Autodesk Inventor part; units mm, degrees
ref_plane "YZ Plane" through (0, 0, 0) normal (1, 0, 0) x (0, 1, 0)
ref_plane "XZ Plane" through (0, 0, 0) normal (0, 1, 0) x (-1, 0, 0)
ref_plane "XY Plane" through (0, 0, 0) normal (0, 0, 1) x (1, 0, 0)
sketch "Sketch1" plane through (0, 0, 0) normal (1, 0, 0) x (0, 1, 0)
  arc A0 (-3.4223, -4.604) -> (-3.4223, -18.104) centre (2.5306, -11.354) ccw
  line L0 (-20.4694, -3.1126) -> (-20.4694, -19.5954)
  line L1 (-3.4223, -18.104) -> (-20.4694, -19.5954)
  line L2 (-3.4223, -4.604) -> (-20.4694, -3.1126)
  point P0 (0, 0)
  dimension "d5" = 23
  dimension "d21" = 9
  dimension "d28" = 85
extrude "Extrusion1" add sketch "Sketch1" along normal blind 14
draft "FaceDraft3" angle 8 pull direction (0, 1, 0) faces at (0, -15.7807, -10.9914) fixed edges at (0, -20.4694, -11.354)
draft "FaceDraft4" angle 8 pull direction (0, 1, 0) faces at (14, -15.7807, -10.9914) fixed edges at (14, -20.4694, -11.354)
properties part number "BaseGarra"
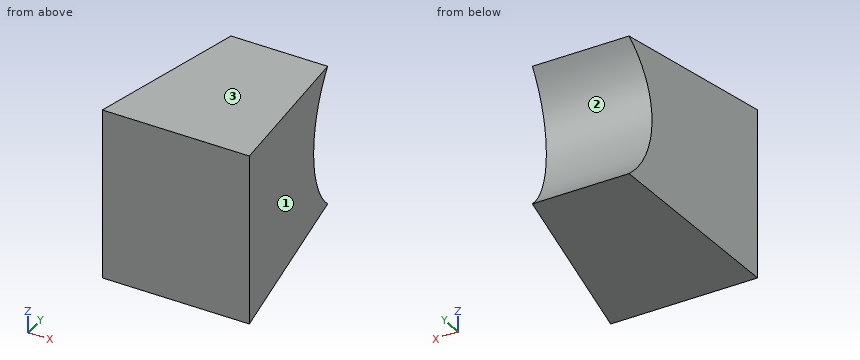
Here's how the part is built. I have some questions about the finished solid (model axes, mm). Face numbers are marked on the shaded views. Give positions to 0.01 mm unless a question says otherwise; leave off trailing zeros. Write each loop counter-clockwise with the first axis right and the second up, starting at its lowest first coordinate (ties: lowest second). Pieces come first, ordered by that corner, then holes. Notation, with made-up numbers: (-10, 45.25) -> (3, 45.25) arc R9 ccw to (3, 51.25) -> close; hole circle Ø2 at (56.5, -19). An arc over 180 degrees is marked (long way). Use one line per item in the form item = value.
1) Suppose I cut it at B-B (x = 8.75). Please give me the cut outline in (y, z).
Verdict:
outline = (-20.47, -19.6) -> (-3.42, -18.1) arc R9 cw to (-3.42, -4.6) -> (-20.47, -3.11) -> close
2) If I drill on L1, parallel to Y at x = 9.75, z = -11.25; L2, parallel to Z at x = 9.5, y = -4.75; L3, parallel to X at y = -17.5, z = -9, over which ranges is the centre line in solid material (lowest first)? Write a range as [from, to].
Verdict:
L1 = [-20.47, -6.47]
L2 = [-18.22, -16.64], [-6.06, -4.49]
L3 = [0.42, 13.58]
3) We'd pull the mould along Z, two halves only. Please class the marked faces 1, 2 and 3: +Z half, -Z half, draft (parallel to the pull), parting line (faces both ways), or undercut.
Verdict:
face_1 = draft
face_2 = undercut
face_3 = +Z half
4) Suppose I cut it at C-C (z = -7). Please give me the cut outline in (x, y).
Verdict:
outline = (0, -20.47) -> (14, -20.47) -> (11.87, -5.35) -> (2.13, -5.35) -> close
5) I'm going to push flat-ended pins straight in: pin 1 (5 mm diameter, centred on x = 9, y = -9.5, fed in from +Z); pin 2 (2 mm diameter, centred on x = 4, y = -5.5, fed in from -Z); pin 3 (1 mm diameter, centred on y = -11, z = -10.5, fed in from -X). Where does each tip first touch, or does it pass through?
Verdict:
pin_1 = -3.85
pin_2 = -18.37
pin_3 = 1.26
6) Suppose I cut it at A-A (y = -5.25). Please give me the cut outline in (x, z), and give its area (3 significant figures).
Verdict:
outline = (2.14, -18.26) -> (11.86, -18.26) -> (11.86, -15.88) -> (2.14, -15.88) -> close; (2.14, -6.83) -> (11.86, -6.83) -> (11.86, -4.44) -> (2.14, -4.44) -> close
area = 46.4 mm2
